Print and shaded views of the part. All mm, measured from the part's lowest x, y and z. Round coordinates to 2 decimals unless told otherwise and drop trailing zeros. Loops run counter-clockwise (first coordinate to the right, second up) from the corner with the lowest first, then second, coordinate; pieces in that order, holes last. Notation, with made-up numbers: M 52.25,-12 L 86.25,-12 A23 cw 86.25,7 Z; hole C 23,18 d2. An arc over 180 degrees is marked long. One line per item, written item: value. Start each with the question number.
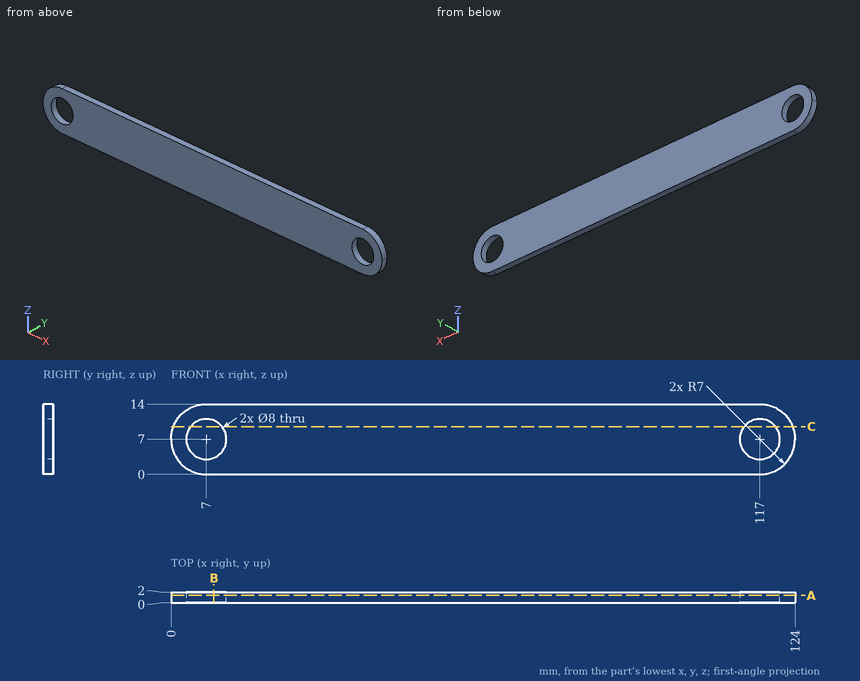
(1) Slice it at C-C, the plane z = 9.5. List the corners of the cut face in (x, y).
(2) Slice it at A-A, the plane y = 1.4. Count the separate pieces of the cut face and the enclosed holes in it, and give its area (3 significant figures).
(3) Slice it at B-B, the plane x = 8.5. List the corners of the cut face in (y, z).
(4) Probe L1, parallel to Z at x = 7, y = 0.5; L2, parallel to Z at x = 116, y = 1.05; L3, parallel to X at y = 0.2, z = 1.25. List the from-to ranges inside material, lowest first.
Check result:
1. outline: M 0.46,0 L 3.88,0 L 3.88,2 L 0.46,2 Z; M 10.12,0 L 113.88,0 L 113.88,2 L 10.12,2 Z; M 120.12,0 L 123.54,0 L 123.54,2 L 120.12,2 Z
2. separate pieces: 1
2. enclosed holes: 2
2. area: 1,590 mm^2
3. outline: M 0,0 L 2,0 L 2,3.29 L 0,3.29 Z; M 0,10.71 L 2,10.71 L 2,14 L 0,14 Z
4. L1: z = 0 to 3, 11 to 14
4. L2: z = 0 to 3.13, 10.87 to 14
4. L3: x = 3.01 to 120.99
